Check sheet for the modelled part. Datum: model origin and axes. Units: mm. Round coordinates to 2 decimals unless told otherwise and drop trailing zeros. Write each loop counter-clockwise with the first axis right and the second up, starting at its lowest first coordinate (ties: lowest second). Pieces come first, ordered by that corner, then holes. Notation, with made-up numbers: (62, -34) -> (103, -34) arc R18 cw to (103, -26) -> close; hole circle Ø8 at (-22.5, 78.25). An arc over 180 degrees is marked (long way). One line per item, written item: value.
from build123d import *

# Parameters (mm, degrees)
F0_R     = 63.453437
F0_R_2   = 1.586336
F1_DEPTH = 19.05


with BuildPart() as f1:
    # F0 (on Top) → F1 (new body)
    with BuildSketch(Plane.XY):
        with Locations((76.21336, 77.152969)):
            Circle(F0_R)
        with Locations((40.325263, 41.264868)):
            Circle(F0_R_2, mode=Mode.SUBTRACT)
        with Locations((76.21336, 26.399533)):
            Circle(F0_R_2, mode=Mode.SUBTRACT)
        with Locations((25.459923, 77.152967)):
            Circle(F0_R_2, mode=Mode.SUBTRACT)
        with Locations((112.101459, 41.26487)):
            Circle(F0_R_2, mode=Mode.SUBTRACT)
        with Locations((126.966796, 77.152967)):
            Circle(F0_R_2, mode=Mode.SUBTRACT)
        with Locations((40.325261, 113.041068)):
            Circle(F0_R_2, mode=Mode.SUBTRACT)
        with Locations((76.21336, 127.906406)):
            Circle(F0_R_2, mode=Mode.SUBTRACT)
        with Locations((112.101461, 113.041067)):
            Circle(F0_R_2, mode=Mode.SUBTRACT)
    extrude(amount=F1_DEPTH)


solid = f1.part
Item 1: Depth check by flat-ended pin: pin 1 (4 mm diameter, centred on x = 69, z = 10, fed in from -Y); pin 2 (2 mm diameter, centred on y = 80, z = 5.5, fed in from -X); pin 3 (10 mm diameter, centred on y = 90, z = 3, fed in from -X); pin 4 (3 mm diameter, centred on x = 112.1, y = 41.26, fed in from -Z). Enter the tip coordinate at first touch or a pass-through.
Result set:
pin 1: y = 13.91
pin 2: x = 12.79
pin 3: x = 13.25
pin 4: through
Item 2: Release check for a two-part mould opening along X. For faces 1 (the cylindrical face through (39.981, 111.492, 9.392)), 2 (the cylindrical face through (26.192, 75.746, 9.392)), 3 (the cylindrical face through (67.953, 140.066, 9.392)), 4 (the flat face through (75, 78, 0)) record: pulls with the +X half, pulls with the -X half, needs draft (parallel to the pull), parting line crosses it, or undercut.
Result set:
face 1: undercut
face 2: undercut
face 3: parting line crosses it
face 4: needs draft
Item 3: Sectioned sample at B-B (x = 94). Enter the section's corners in (y, z).
Result set:
outline: (16.24, 0) -> (138.06, 0) -> (138.06, 19.05) -> (16.24, 19.05) -> close
Item 4: Material ranges on line 1 along Y through (x, z) = (76, 3); line 2 along Y through (x, z) = (39.5, 5); line 3 along X through (y, z) = (83, 6.75), recorded low to high.
Result set:
line 1: 13.7 to 24.83, 27.97 to 126.33, 129.48 to 140.61
line 2: 25.4 to 39.91, 42.62 to 111.69, 114.4 to 128.91
line 3: 13.03 to 139.4
Item 5: Sectioned sample at C-C (y = 105). Enter the section's corners in (x, z), then the cut area to 3 significant figures.
Result set:
outline: (19.2, 0) -> (133.23, 0) -> (133.23, 19.05) -> (19.2, 19.05) -> close
area: 2,170 mm^2
Item 6: Sectioned sample at A-A (z = 12.25). State how many separate pieces and enclosed holes the cut face has, then the cut area to 3 significant figures.
Result set:
separate pieces: 1
enclosed holes: 8
area: 12,600 mm^2
